Source: three-view drawing plus pictorial views. Frame: mm from the lowest corner of the part. Give positions to 0.01 mm unless a question says otherwise; leave off trailing zeros. Write each loop counter-clockwise with the first axis right and the second up, starting at its lowest first coordinate (ties: lowest second). Pieces come first, ordered by that corner, then holes. Notation, with made-up numbers: M 8,0 L 44,0 A28 cw 44,21 Z; hole C -39,-12.5 d10. An arc over 180 degrees is marked long. One line per question, with ' | ' between items.
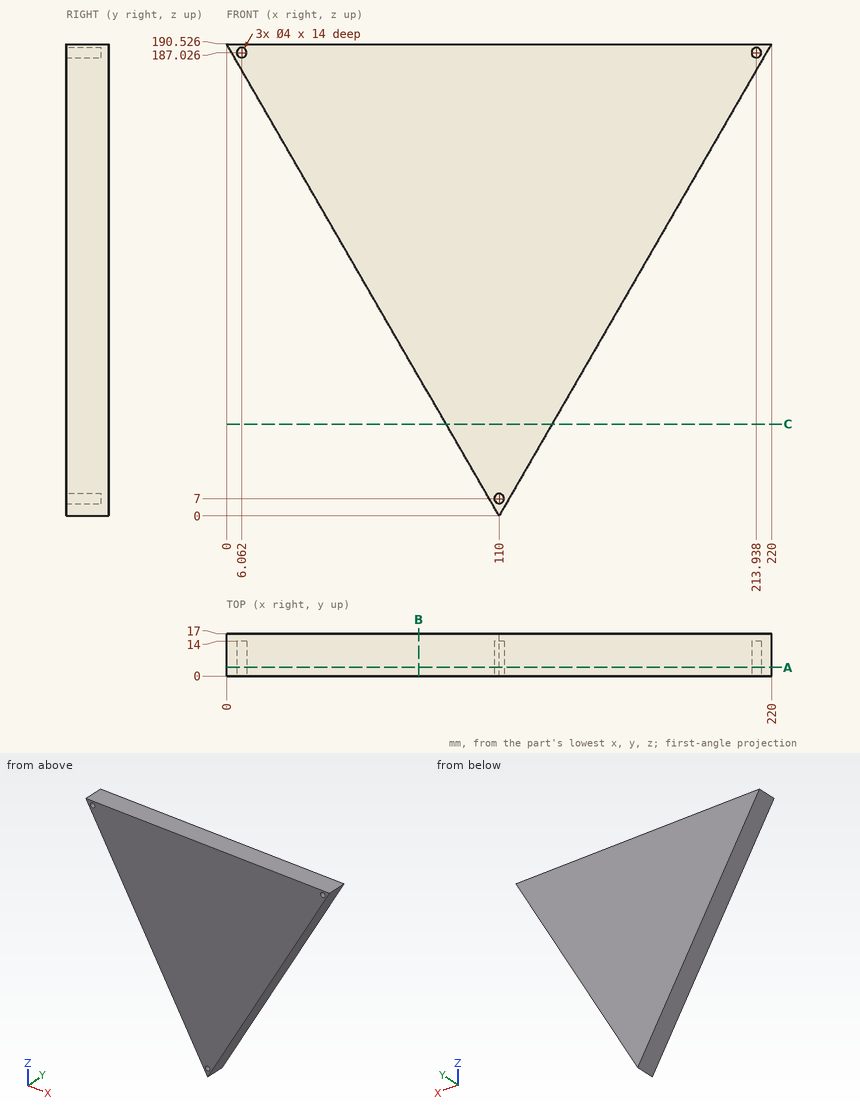
(1) Material intervals for L1, parallel to Z at x = 110, y = 6.5 (1 decimal); L2, parallel to X at y = 3, z = 7; L3, parallel to Z at x = 195.5, y = 4 (1 decimal), sorted ascending. Write a range as [from, to].
Working result:
L1: z = [0, 5], [9, 190.5] | L2: x = [105.96, 108], [112, 114.04] | L3: z = [148.1, 190.5]
(2) Cut plane A-A, the plane y = 3.5. Return loops of the section in (x, z) (1 decimal), then the cut area to 3 significant figures.
Working result:
outline: M 0,190.5 L 110,0 L 220,190.5 Z; hole C 6.1,187 d4; hole C 110,7 d4; hole C 213.9,187 d4 | area: 20,900 mm^2
(3) Cut plane C-C, the plane z = 37. Return loops of the section in (x, y).
Working result:
outline: M 88.64,0 L 131.36,0 L 131.36,17 L 88.64,17 Z
(4) Cut plane B-B, the plane x = 77.5. Return loops of the section in (y, z) (1 decimal), then the cut area to 3 significant figures.
Working result:
outline: M 0,56.3 L 17,56.3 L 17,190.5 L 0,190.5 Z | area: 2,280 mm^2
(5) First-contact query: P1, Ø1, axis at y = 2, z = 95, coming from the -X side; P2, Ø10, axis at y = 13.5, z = 104.5, coming from the -X side; P3, Ø1.5, axis at y = 7, z = 167.5, coming from the +X side. Flat tips, straight axial feed; report the tip coordinate or a pass-through.
Working result:
P1: stops at x = 54.86 | P2: stops at x = 46.78 | P3: stops at x = 207.14
